Part model, mm, in its own coordinate system. A direction names the side the tool comes from. Coordinates: 2 decimals unless noted, no trailing zeros. Loops run counter-clockwise (first coordinate to the right, second up) from the corner with the lowest first, then second, coordinate; pieces in that order, holes last. Notation, with made-up numbers: (64, 7) - (114, 7) arc R10 cw to (114, 20) - close; hole circle Ø3 at (23.25, -35). An arc over 180 degrees is marked (long way). Answer as CSV lines item,"result".
from build123d import *

# Parameters (mm, degrees)
CROQUIS1_W              = 74
CROQUIS1_H              = 46.3
CROQUIS1_R              = 17
CROQUIS1_R_2            = 2.1
SALIENTE_EXTRUIR1_DEPTH = 4
SALIENTE_EXTRUIR3_DEPTH = 74
CORTAR_EXTRUIR2_REACH   = 12.65
CROQUIS6_R              = 3.25


with BuildPart() as part:
    # Croquis1 → Saliente-Extruir1 (new body)
    with BuildSketch(Plane.XY):
        with Locations((0, -2)):
            Rectangle(CROQUIS1_W, CROQUIS1_H)
        Circle(CROQUIS1_R, mode=Mode.SUBTRACT)
        with Locations((-15.5, -15.5)):
            Circle(CROQUIS1_R_2, mode=Mode.SUBTRACT)
        with Locations((-15.5, 15.5)):
            Circle(CROQUIS1_R_2, mode=Mode.SUBTRACT)
        with Locations((15.5, -15.5)):
            Circle(CROQUIS1_R_2, mode=Mode.SUBTRACT)
        with Locations((15.5, 15.5)):
            Circle(CROQUIS1_R_2, mode=Mode.SUBTRACT)
    extrude(amount=SALIENTE_EXTRUIR1_DEPTH)

    # Croquis5 → Saliente-Extruir3 (add)
    with BuildSketch(Plane.ZY.offset(37)):
        Polygon((4, -25.15), (62, -25.15), (62, -14.5), (40, -14.5), (40, -21.85), (4, -21.85), align=None)
    extrude(amount=-SALIENTE_EXTRUIR3_DEPTH)

    # Croquis6 → Cortar-Extruir2 (cut, up to next)
    with BuildSketch(Plane(origin=(0, -14.5, 0), x_dir=(1, 0, 0), z_dir=(0, 1, 0)), mode=Mode.PRIVATE) as cortar_extruir2_sk1:
        with Locations((-30, -51)):
            Circle(CROQUIS6_R)
    cortar_extruir2_tool1 = extrude(cortar_extruir2_sk1.sketch, amount=-CORTAR_EXTRUIR2_REACH, mode=Mode.PRIVATE) & part.part
    add(cortar_extruir2_tool1.solids().sort_by_distance((-30, -14.5, 51))[0], mode=Mode.SUBTRACT)
    # Croquis6 → Cortar-Extruir2 (cut, up to next)
    with BuildSketch(Plane(origin=(0, -14.5, 0), x_dir=(1, 0, 0), z_dir=(0, 1, 0)), mode=Mode.PRIVATE) as cortar_extruir2_sk2:
        with Locations((30, -51)):
            Circle(CROQUIS6_R)
    cortar_extruir2_tool2 = extrude(cortar_extruir2_sk2.sketch, amount=-CORTAR_EXTRUIR2_REACH, mode=Mode.PRIVATE) & part.part
    add(cortar_extruir2_tool2.solids().sort_by_distance((30, -14.5, 51))[0], mode=Mode.SUBTRACT)


solid = part.part
Q1. Saw through at B-B (z = 51). Give the cut face in (x, y), then the cut area to 3 significant figures.
Results:
outline,"(-37, -25.15) - (-33.25, -25.15) - (-33.25, -14.5) - (-37, -14.5) - close; (-26.75, -25.15) - (26.75, -25.15) - (26.75, -14.5) - (-26.75, -14.5) - close; (33.25, -25.15) - (37, -25.15) - (37, -14.5) - (33.25, -14.5) - close"
area,"650 mm^2"
Q2. Two-plate mould, pull along Y, no slides. Class faces 1 (the face through (-17, -7, 0)), 2 (the face through (-14.37, 17.27, 1.97)), 3 (the face through (-1, -21.85, 22)): released by +Y, released by -Y, zero draft, split by the parting line, or undercut.
Results:
face 1,"zero draft"
face 2,"undercut"
face 3,"released by +Y"
Q3. Wall check: L1, parallel to Y at x = 0, z = 2; L2, parallel to X at y = -15, z = 1; L3, parallel to Z at x = 27.5, y = 2. Give the ranges that are in metal, low to high.
Results:
L1,"y = -25.15 to -17, 17 to 21.15"
L2,"x = -37 to -17.54, -13.46 to -8, 8 to 13.46, 17.54 to 37"
L3,"z = 0 to 4"
Q4. Saw through at A-A (x = 0). Give the cut face in (y, z), then the cut area to 3 significant figures.
Results:
outline,"(-25.15, 0) - (-17, 0) - (-17, 4) - (-21.85, 4) - (-21.85, 40) - (-14.5, 40) - (-14.5, 62) - (-25.15, 62) - close; (17, 0) - (21.15, 0) - (21.15, 4) - (17, 4) - close"
area,"402 mm^2"
Q5. Saw through at C-C (y = 0). Give the cut face in (x, z).
Results:
outline,"(-37, 0) - (-17, 0) - (-17, 4) - (-37, 4) - close; (17, 0) - (37, 0) - (37, 4) - (17, 4) - close"
Q6. Saw through at D-D (y = -15.5). Give the cut face in (x, z).
Results:
outline,"(-37, 0) - (-17.6, 0) - (-17.6, 4) - (-37, 4) - close; (-37, 40) - (37, 40) - (37, 62) - (-37, 62) - close; (-13.4, 0) - (-6.98, 0) - (-6.98, 4) - (-13.4, 4) - close; (6.98, 0) - (13.4, 0) - (13.4, 4) - (6.98, 4) - close; (17.6, 0) - (37, 0) - (37, 4) - (17.6, 4) - close; hole circle Ø6.5 at (-30, 51); hole circle Ø6.5 at (30, 51)"
Q7. Flat gauge pins, fed straight in: pin 1 (8.5 mm diameter, centred on x = -30, z = 51, fed in from +Y); pin 2 (6 mm diameter, centred on x = -26.5, z = 28.5, fed in from +Y); pin 3 (20.5 mm diameter, centred on x = 0, y = 0, fed in from -Z); pin 4 (1 mm diameter, centred on x = 19, y = 10.5, fed in from +Z). Where does each tip first touch, or does it go through?
Results:
pin 1,"stops at y = -14.5"
pin 2,"stops at y = -21.85"
pin 3,"passes through"
pin 4,"stops at z = 4"
Q8. Which spindle directions (+Z, -Z, +X, -X, +Y, -Y) get a long thin tool onto all of the face, cutting with end or side? Do faces 4 (the face through (-17, -5, 4)), 5 (the face through (37, -22.5, 26.3)), 6 (the face through (9.139, 14.334, 1.972)), 7 (the face through (-37, -22.5, 26.3)), 8 (the face through (-1, -14.5, 51)). Say none if no direction does.
Results:
face 4,"+X, -X, +Y"
face 5,"+Z, -Z, +X, +Y, -Y"
face 6,"-Z"
face 7,"+Z, -Z, -X, +Y, -Y"
face 8,"+Z, +X, -X, +Y"
